Job drawing, mm, ordinate dimensions from the low corner. One solid piece. A direction names the side the tool comes from. Round coordinates to 2 decimals unless told otherwise and drop trailing zeros. Write each loop counter-clockwise with the first axis right and the second up, starting at its lowest first coordinate (ties: lowest second). Pieces come first, ordered by that corner, then holes. Notation, with made-up numbers: M 9,34 L 52,34 A8 ccw 52,44 Z; hole C 5,62.25 d7. An arc over 180 degrees is marked long. Answer as a JSON object with one key per item and string values. Group by question number.
1. Band-saw the part on C-C, the plane y = 8. Write the cut outline in (x, z), plus the area to 3 significant figures.
2. Drop flat-ended pins along their axis: pin 1 (2 mm diameter, centred on x = 1.5, y = 12.5, fed in from +Z); pin 2 (0.6 mm diameter, centred on x = 2, z = 4, fed in from +Y). Give the stop position or say it passes through.
3. Band-saw the part on B-B, the plane y = 14.5. Write the cut outline in (x, z), plus the area to 3 significant figures.
4. Drill centre lines: line 1 (X direction, y = 12, z = 2.1); line 2 (Z direction, x = 1.6, y = 8); line 3 (X direction, y = 4.25, z = 3.3). Where is each one in solid material? Low to high. Write a range as from..to.
5. Which spindle directions (+Z, -Z, +X, -X, +Y, -Y) get a long thin tool onto all of the face, cutting with end or side? Do the marked faces 1, 2 and 3. Say none if no direction does.
6. Band-saw the part on A-A, the plane x = 2. Write the cut outline in (y, z), plus the area to 3 significant figures.
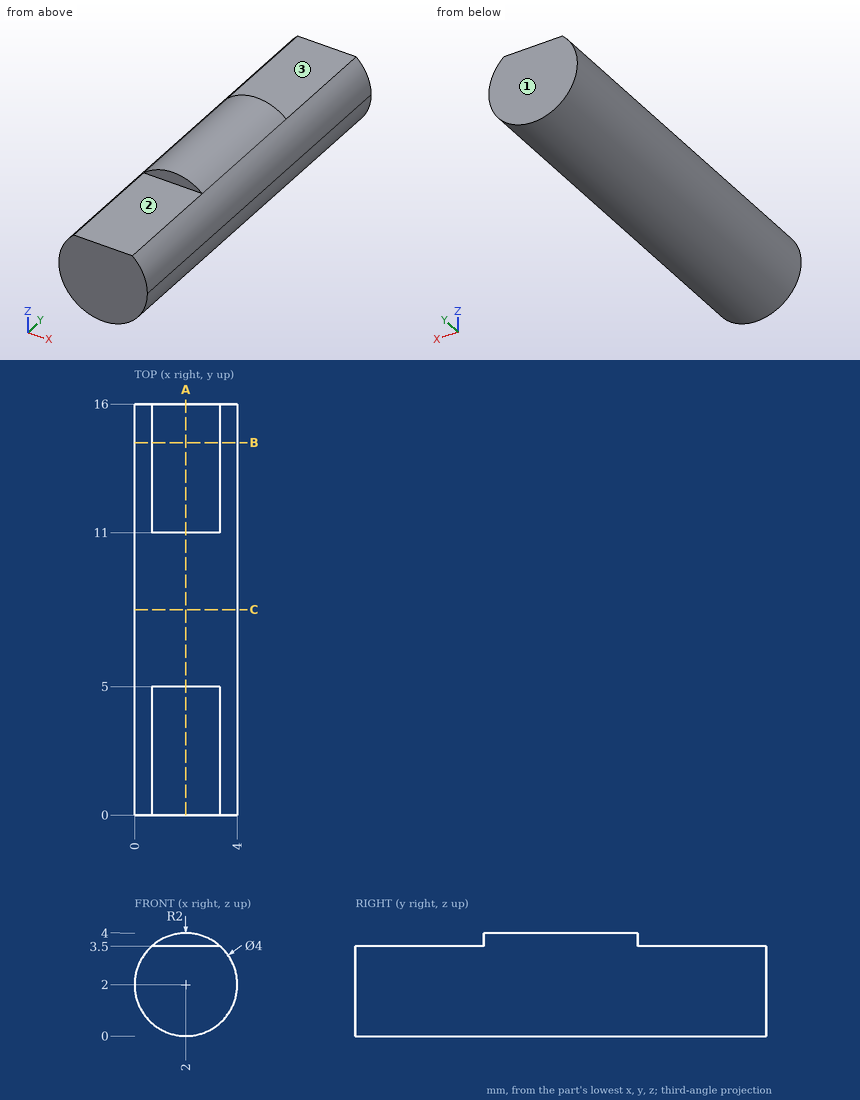
Worked answers:
{
 "1": {"outline": "C 2,2 d4", "area": "12.6 mm^2"},
 "2": {"pin 1": "stops at z = 3.5", "pin 2": "stops at y = 11"},
 "3": {"outline": "M 0.68,3.5 A2 ccw long 3.32,3.5 Z", "area": "11.7 mm^2"},
 "4": {"line 1": "x = 0..4", "line 2": "z = 0.04..3.96", "line 3": "x = 0.48..3.52"},
 "5": {"face 1": "+Z, -Z, +X, -X, +Y", "face 2": "+Z, +X, -X, -Y", "face 3": "+Z, +X, -X, +Y"},
 "6": {"outline": "M 0,0 L 16,0 L 16,3.5 L 11,3.5 L 11,4 L 5,4 L 5,3.5 L 0,3.5 Z", "area": "59.0 mm^2"}
}
